The figure shows three views and two pictorial views of one solid part (mm, origin at its lowest corner). Answer the questions. A direction names the side the tool comes from. Round coordinates to 2 decimals unless told otherwise and drop trailing zeros. Loops run counter-clockwise (first coordinate to the right, second up) from the corner with the lowest first, then second, coordinate; pieces in that order, holes last. Notation, with made-up numbers: (-10.75, -28) -> (8.25, -28) arc R23 ccw to (8.25, 11) -> close; hole circle Ø3 at (79.5, 33.25). An arc over 180 degrees is marked (long way). Put each result on its own line as item: value.
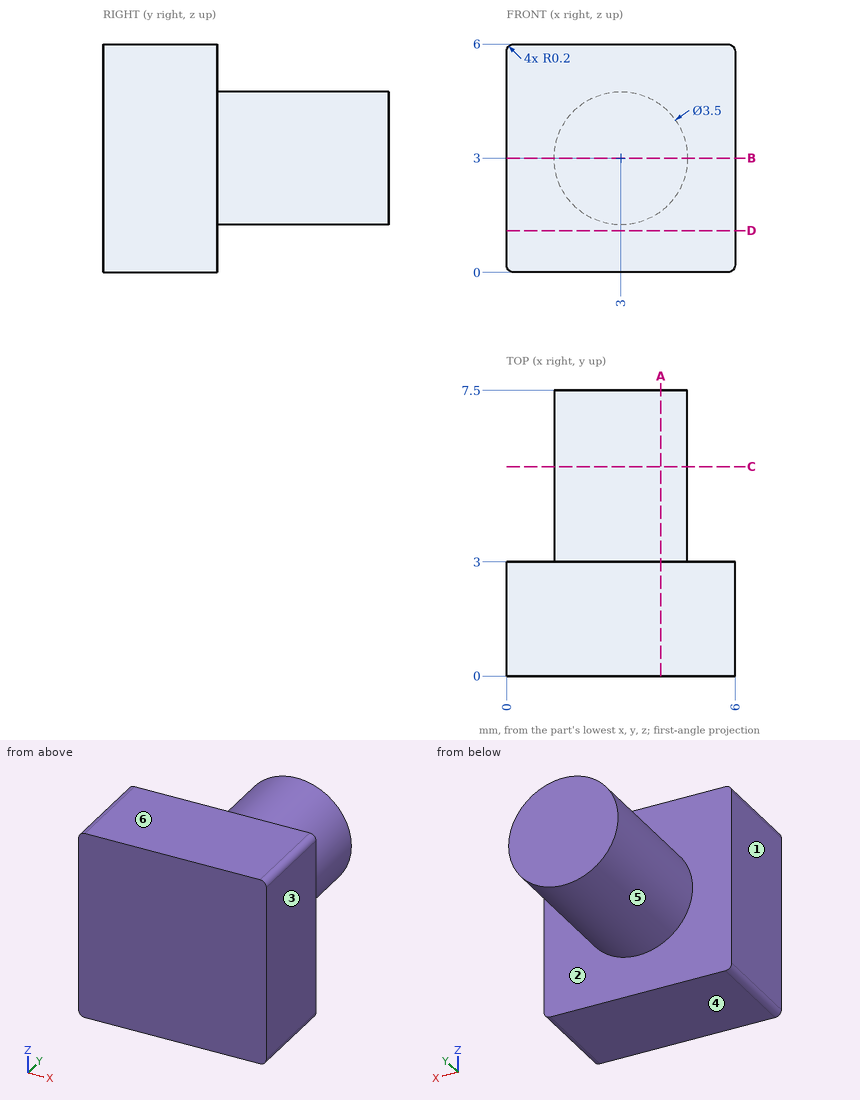
Item 1: The part is cut by section D-D (z = 1.1). Determine the outline of the cut face in (x, y), then the cut area to 3 significant figures.
Derived:
outline: (0, 0) -> (6, 0) -> (6, 3) -> (0, 3) -> close
area: 18.0 mm^2
Item 2: The part is cut by section A-A (x = 4.05). Determine the outline of the cut face in (y, z), then the cut area to 3 significant figures.
Derived:
outline: (0, 0) -> (3, 0) -> (3, 1.6) -> (7.5, 1.6) -> (7.5, 4.4) -> (3, 4.4) -> (3, 6) -> (0, 6) -> close
area: 30.6 mm^2
Item 3: The part is cut by section B-B (z = 3). Determine the outline of the cut face in (x, y).
Derived:
outline: (0, 0) -> (6, 0) -> (6, 3) -> (4.75, 3) -> (4.75, 7.5) -> (1.25, 7.5) -> (1.25, 3) -> (0, 3) -> close
Item 4: Flat-ended cylindrical pins translate along their axes: pin 1 Ø3 at (x, y) = (4.5, 6) entering from -Z; pin 2 Ø1.5 at (y, z) = (2.5, 3.5) entering from -X; pin 3 Ø1.5 at (y, z) = (6, 1) entering from -X; pin 4 Ø1 at (x, z) = (0.5, 4) entering from +Y. Find the tip coordinate at first contact, or state that the pin passes through.
Derived:
pin 1: stops at z = 1.25
pin 2: stops at x = 0
pin 3: stops at x = 1.78
pin 4: stops at y = 3
Item 5: For a pull along Z with two mould halves and no side action, classify the marked faces 3, 4, 5 and 6 as pulls with the +Z half, pulls with the -Z half, needs draft (parallel to the pull), parting line crosses it, or undercut.
Derived:
face 3: needs draft
face 4: pulls with the -Z half
face 5: parting line crosses it
face 6: pulls with the +Z half
Item 6: Which of the six approach directions +Z, -Z, +X, -X, +Y, -Y give full straight-line access (tool end or side, diameter ignored) to the marked faces 1 and 2?
Derived:
face 1: +Z, -Z, -X, +Y, -Y
face 2: +Y
Item 7: Find the intervals of material crossed by line 1 along Y through (x, z) = (4.95, 2.8); line 2 along Z through (x, y) = (4.4, 7.25); line 3 along Z through (x, y) = (3.15, 4.25), in increasing order.
Derived:
line 1: y = 0 to 3
line 2: z = 1.95 to 4.05
line 3: z = 1.26 to 4.74
Item 8: The part is cut by section C-C (y = 5.5). Determine the outline of the cut face in (x, z).
Derived:
outline: circle Ø3.5 at (3, 3)
